from build123d import *

# Parameters (mm, degrees)
SKETCH1_W           = 20
SKETCH1_H           = 200
BOSS_EXTRUDE1_DEPTH = 20
SKETCH4_R           = 22.5
BOSS_EXTRUDE3_DEPTH = 10


with BuildPart() as part:
    # Sketch1 → Boss-Extrude1 (new body)
    with BuildSketch(Plane.XY):
        Rectangle(SKETCH1_W, SKETCH1_H)
    extrude(amount=BOSS_EXTRUDE1_DEPTH)

    # Sketch4 → Boss-Extrude3 (add)
    with BuildSketch(Plane(origin=(0, 100, 0), x_dir=(1, 0, 0), z_dir=(0, 1, 0))):
        with Locations(Location((0, -10, 0), (0, 0, 270))):
            Circle(SKETCH4_R)
    extrude(amount=-BOSS_EXTRUDE3_DEPTH)


solid = part.part
Can you work these out from the model? Positions are in its coordinate system, mm. A direction names the side the tool comes from. Give positions to 0.01 mm unless a question says otherwise; leave off trailing zeros. Loops run counter-clockwise (first coordinate to the right, second up) from the corner with the lowest first, then second, coordinate; pieces in that order, holes last. Notation, with made-up numbers: M -40,0 L 8,0 A30 cw 8,34 Z; hole C 13,-7 d4. An arc over 180 degrees is marked long. One line per item, written item: value. Start each with the question number.
1) If we section it at A-A, the plane z = 10: Write out the boundary of the cut face in (x, y), and give its area (3 significant figures).
2) If we section it at B-B, the plane x = 0: Write out the boundary of the cut face in (y, z).
3) If we section it at C-C, the plane y = 34: Write out the boundary of the cut face in (x, z).
4) I'm going to push flat-ended pins straight in: pin 1 (3 mm diameter, centred on y = 68, z = 17, fed in from -X); pin 2 (1 mm diameter, centred on x = 3, y = -1, fed in from -Z); pin 3 (6 mm diameter, centred on y = 33.5, z = 9.5, fed in from +X). Where does each tip first touch, or does it pass through?
5) On a 3-axis mill with a long thin cutter (end or side, diameter ignored), from which of +Z, -Z, +X, -X, +Y, -Y can I reach the whole of each face in a straight line? I mean faces 1 (the face through (10, -6, 10)), 2 (the face through (0, -4, 20)), 3 (the face through (-10, -6, 10)), 4 (the face through (0, -100, 10)), 5 (the face through (0, -4, 0)). Say none if no direction works.
6) If we section it at D-D, the plane x = 18: Write out the boundary of the cut face in (y, z), and give its area (3 significant figures).
7) If I drill on line 1 (Z direction, x = -4, y = 44); line 2 (X direction, y = -82, z = 12.5); line 3 (Y direction, x = 20.5, z = 4), over which ranges is the centre line in solid material (lowest first)? Write a range as [from, to].
Completed:
1. outline: M -22.5,90 L -10,90 L -10,-100 L 10,-100 L 10,90 L 22.5,90 L 22.5,100 L -22.5,100 Z
1. area: 4,250 mm^2
2. outline: M -100,0 L 90,0 L 90,-12.5 L 100,-12.5 L 100,32.5 L 90,32.5 L 90,20 L -100,20 Z
3. outline: M -10,0 L 10,0 L 10,20 L -10,20 Z
4. pin 1: stops at x = -10
4. pin 2: stops at z = 0
4. pin 3: stops at x = 10
5. face 1: +Z, -Z, +X, -Y
5. face 2: +Z, +X, -X, -Y
5. face 3: +Z, -Z, -X, -Y
5. face 4: +Z, -Z, +X, -X, -Y
5. face 5: -Z, +X, -X, -Y
6. outline: M 90,-3.5 L 100,-3.5 L 100,23.5 L 90,23.5 Z
6. area: 270 mm^2
7. line 1: z = [0, 20]
7. line 2: x = [-10, 10]
7. line 3: y = [90, 100]
